Could you check a few things on this model? Use its own coordinates, in mm. A direction names the side the tool comes from. Round coordinates to 2 decimals unless told otherwise and drop trailing zeros. Write each loop counter-clockwise with the first axis right and the second up, starting at its lowest first coordinate (ties: lowest second). Pieces come first, ordered by that corner, then holes. Notation, with made-up numbers: (82.25, -10) -> (117.25, -10) arc R17 cw to (117.25, 21) -> close; hole circle Ø4 at (44, 23.25). An arc over 180 degrees is marked (long way). Answer in a Markdown table with one row per item.
Autodesk Inventor part; units mm, degrees
ref_plane "YZ Plane" through (0, 0, 0) normal (1, 0, 0) x (0, 1, 0)
ref_plane "XZ Plane" through (0, 0, 0) normal (0, 1, 0) x (-1, 0, 0)
ref_plane "XY Plane" through (0, 0, 0) normal (0, 0, 1) x (1, 0, 0)
sketch "Эскиз1" plane through (0, 0, 0) normal (0, 0, 1) x (1, 0, 0)
  line L0 (0, 0) -> (0, 190)
  line L1 (0, 190) -> (110, 190)
  line L2 (110, 190) -> (110, 240)
  line L3 (110, 240) -> (152, 240)
  line L4 (152, 240) -> (152, 290)
  line L5 (152, 290) -> (187, 290)
  line L6 (187, 290) -> (187, 190)
  line L7 (0, 190) -> (0, 160)
  line L8 (0, 160) -> (268.4083, 160)
  line L9 (187, 190) -> (218.141, 190) construction
  line L10 (187, 190) -> (157, 160)
  line L11 (0, 160) -> (30, 160)
  line L12 (30, 160) -> (30, 70)
  line L13 (30, 70) -> (70, 70)
  line L14 (70, 70) -> (70, 0)
  line L15 (70, 0) -> (45, 0)
  line L16 (45, 0) -> (45, 45.5)
  line L17 (45, 45.5) -> (0, 45.5)
  line L18 (120, 240) -> (120, 232)
  line L19 (120, 232) -> (128, 232)
  line L20 (128, 232) -> (128, 240)
  dimension "d0" = 190
  dimension "d1" = 110
  dimension "d2" = 50
  dimension "d3" = 42
  dimension "d4" = 50
  dimension "d5" = 35
  dimension "d6" = 100
  dimension "d9" = 30
  dimension "d12" = 45
  dimension "d13" = 30
  dimension "d14" = 90
  dimension "d15" = 40
  dimension "d16" = 25
  dimension "d17" = 45.5
  dimension "d35" = 8
  dimension "d36" = 8
  dimension "d54" = 10
revolve "Вращение1" add sketch "Эскиз1" angle 360 about axis through (70, 0, 0) along (-1, 0, 0) contours L0 L8 L12 L13 L14 L15 L16 L17 | L0 L1 L2 L3 L18 L19 L20 L4 L5 L6 L10 L8
sketch "Эскиз2" plane through (0, 0, 0) normal (0, 0, 1) x (1, 0, 0)
  line L0 (30, -160) -> (30, 160)
  line L1 (30, 70) -> (70, 70)
  line L2 (157, 160) -> (30, 160)
  line L3 (30, -70) -> (30, 70)
  line L4 (30, 70) -> (30, 65)
  line L5 (30, 65) -> (90, 65)
  line L6 (90, 65) -> (157, 160)
  point P0 (0, 0)
  dimension "d25" = 5
  dimension "d26" = 60
extrude "Выдавливание1" add sketch "Эскиз2" along normal mid plane 15
pattern_circular "Круговой массив1" count 6 over 360 about axis through (169.5, 0, 0) along (1, 0, 0) of "Выдавливание1"
sketch "Эскиз6" plane through (0, 0, 0) normal (0, 1, 0) x (-1, 0, 0)
  line L0 (0, -190) -> (-110, -190)
  line L1 (0, 190) -> (0, -190)
  line L2 (37.4, 0) -> (-224.4, 0)
  line L3 (0, -190) -> (-110, -190)
  line L4 (-49.2747, -190) -> (0, -176)
  point P0 (0, 0)
revolve "Вращение2" cut sketch "Эскиз6" angle 30 mid plane about axis through (169.5, 0, 0) along (1, 0, 0)
pattern_circular "Круговой массив2" count 2 over 360 about axis through (169.5, 0, 0) along (1, 0, 0) of "Вращение2"
sketch "Эскиз7" plane through (187, 0, 0) normal (1, 0, 0) x (0, 0, -1)
  circle A0 centre (0, 0) radius 290
  line L0 (290, 0) -> (265, 0)
  dimension "d43" = 25
hole "Отверстие1" at (187, 0, -265) direction (-1, 0, 0) diameter 26 end through all
pattern_circular "Круговой массив3" count 16 over 360 about axis through (-10, 0, 0) along (1, 0, 0) of "Отверстие1"
properties part number "Крышка цилиндра 1" material "Чугун, серый"
1) Imagine slicing it at A-A, the plane z = 265. Please give me the cut outline in (x, y), plus the area to 3 significant figures.
Findings:
| item | result |
|---|---|
| outline | (152, -117.79) -> (187, -117.79) -> (187, -13) -> (152, -13) -> close; (152, 13) -> (187, 13) -> (187, 117.79) -> (152, 117.79) -> close |
| area | 7,340 mm^2 |
2) Imagine slicing it at D-D, the plane x = 11. Please give me the cut outline in (y, z).
Findings:
| item | result |
|---|---|
| outline | (-49.18, -183.53) -> (-46.36, -173.02) arc R179.13 ccw to (46.36, -173.02) -> (49.18, -183.53) arc R190 ccw to (49.18, 183.53) -> (46.36, 173.02) arc R179.13 ccw to (-46.36, 173.02) -> (-49.18, 183.53) arc R190 ccw to start; hole circle Ø91 at (0, 0) |
3) For pin 1 (2 mm diameter, centred on x = 102.5, z = 156.5, fed in from +Y); pin 2 (4 mm diameter, centred on x = 155.5, z = 174.5, fed in from +Y); pin 3 (6 mm diameter, centred on x = 30, z = -90.5, fed in from -Y), each with a flat end and sliding along its axis, tell me the tip position at first contact or that it passes through.
Findings:
| item | result |
|---|---|
| pin 1 | stops at y = 109.18 |
| pin 2 | stops at y = 233.12 |
| pin 3 | stops at y = -168.65 |
4) Please list where these lines run through material, in increasing order: line 1 (Y direction, x = 107, z = 118); line 2 (Y direction, x = 60, z = -98.5); line 3 (Z direction, x = 119, y = 53).
Findings:
| item | result |
|---|---|
| line 1 | y = -148.92 to -108.06, -76.79 to -59.47, 59.47 to 76.79, 108.06 to 148.92 |
| line 2 | y = -162.47 to -126.09, -65.53 to -48.21, 48.21 to 65.53, 126.09 to 162.47 |
| line 3 | z = -234.07 to -150.97, -106.8 to -91.94, 91.94 to 106.8, 150.97 to 234.07 |
5) For faces 1 (the face through (169.745, 276.608, 87.108)), 2 (the face through (110, 177, -72)), 3 (the face through (94.39, -139.15, -78.98)), which set-ups out of +Z, -Z, +X, -X, +Y, -Y let a thin tool reach every point of the face, with its end or its side?
Findings:
| item | result |
|---|---|
| face 1 | +X, -X |
| face 2 | -X |
| face 3 | +X |
